Here's how the part is built. I have some questions about the finished solid (model axes, mm). A direction names the side the tool comes from. Coordinates: 2 decimals unless noted, no trailing zeros. Loops run counter-clockwise (first coordinate to the right, second up) from the corner with the lowest first, then second, coordinate; pieces in that order, holes last. Notation, with made-up numbers: (-24.5, 17.25) -> (4.5, 17.25) arc R20 cw to (4.5, 46.25) -> close; hole circle Ø6 at (26.5, 28.5). An arc over 180 degrees is marked (long way). Answer as a JSON object with one key per item and string values. Group by question number.
1) Which directions (+Z, -Z, +X, -X, +Y, -Y) give clear straight access to the entire face, cutting with the end or side of a thin tool? Please do faces 5 (the flat face through (6.875, 52, 32)), 6 (the cylindrical face through (-0.325, 100.604, 63.986)).
2) I want a section at A-A (x = -5.5). Write out the boundary of the cut face in (y, z), then the cut area to 3 significant figures.
3) I'm going to push flat-ended pins straight in: pin 1 (6 mm diameter, centred on x = -3.5, z = 29, fed in from +Y); pin 2 (4 mm diameter, centred on x = 5, z = 16.5, fed in from -Y); pin 3 (2.5 mm diameter, centred on x = 1, y = 97.5, fed in from +Z). Where does each tip first touch, or does it pass through?
4) I want a section at B-B (z = 27.5). Write out the boundary of the cut face in (x, y) (3 decimals), then the cut area to 3 significant figures.
5) If we mould it in two halves opening along X, with no side actions, what happens to faces 1 (the flat face through (-6.875, 53, 32)), 2 (the cylindrical face through (0, 0, 32)), 3 (the flat face through (0, 98, 63)), 4 (the flat face through (0, 52, 0))? For each: +X half, -X half, draft (parallel to the pull), parting line (faces both ways), or undercut.
6) I need wall thicknesses on probe 1 along Y at (x, z) = (0, 63.6) (3 decimals); probe 2 along Y at (x, z) = (-5.75, 39); probe 3 along Y at (x, z) = (6, 48.5). Which ranges of each line are inside material? Lowest first, please. Write a range as [from, to].
```python
from build123d import *

# Parameters (mm, degrees)
SKETCH_R     = 2.5
PAD_DEPTH    = 65
SKETCH001_R  = 2.5
PAD001_DEPTH = 63


with BuildPart() as part:
    # Sketch → Pad (new body)
    with BuildSketch(Plane.XY):
        with BuildLine():
            ThreePointArc((-6.875, 6.875), (0, 0), (6.875, 6.875))
            Line((6.875, 6.875), (6.875, 98.125))
            ThreePointArc((6.875, 98.125), (0, 105), (-6.875, 98.125))
            Line((-6.875, 98.125), (-6.875, 6.875))
        make_face()
        with Locations((0, 98.125)):
            Circle(SKETCH_R, mode=Mode.SUBTRACT)
    extrude(amount=PAD_DEPTH)

    # Sketch001 (on Face6 of Pad) → Pad001 (join)
    with BuildSketch(Plane(origin=(0, 0, 0), x_dir=(1, 0, 0), z_dir=(0, 0, -1))):
        with Locations((0, -98.125)):
            Circle(SKETCH001_R)
    extrude(amount=-PAD001_DEPTH)


solid = part.part
```
Determined:
{
 "1": {"face 5": "+Z, -Z, +X, +Y, -Y", "face 6": "+Z"},
 "2": {"outline": "(2.75, 0) -> (102.25, 0) -> (102.25, 65) -> (2.75, 65) -> close", "area": "6,470 mm^2"},
 "3": {"pin 1": "y = 104.98", "pin 2": "y = 0.69", "pin 3": "z = 63"},
 "4": {"outline": "(-6.875, 6.875) arc R6.875 ccw to (6.875, 6.875) -> (6.875, 98.125) arc R6.875 ccw to (-6.875, 98.125) -> close", "area": "1,400 mm^2"},
 "5": {"face 1": "-X half", "face 2": "parting line", "face 3": "undercut", "face 4": "draft"},
 "6": {"probe 1": "[0, 95.625], [100.625, 105]", "probe 2": "[3.11, 101.89]", "probe 3": "[3.52, 101.48]"}
}
